Input: dimensioned drawing with shaded views. Units: mm. Origin: part minimum x, y, z. Round coordinates to 2 decimals unless told otherwise and drop trailing zeros. Order: outer loops, then holes, each group sorted by start corner. A loop starts at its lowest first (then second) coordinate and runs counter-clockwise, first axis right, second up. Notation, with made-up numbers: M -13,36 L -9,36 A5 ccw -9,42 Z; hole C -22.5,4 d8. An arc over 180 degrees is marked long. Answer as CSV lines item,"result". Start each with the question number.
Item 1: First-contact query: P1, Ø12, axis at y = 8.5, z = 10, coming from the +X side (1 decimal); P2, Ø10, axis at y = 16.5, z = 12, coming from the +X side (1 decimal); P3, Ø1, axis at y = 31, z = 19, coming from the -X side; P4, Ø10, axis at x = 8.5, y = 20.5, coming from the -Z side. Flat tips, straight axial feed; report the tip coordinate or a pass-through.
Item 2: Section query B-B on z = 18.5. Return the cut outline in (x, y) (1 decimal).
Item 3: Line query: line 1 (Y direction, x = 8.5, z = 23) (1 decimal); line 2 (Y direction, x = 9, z = 13.75); line 3 (Z direction, x = 12, y = 30.5) (1 decimal). Output: solid intervals per line, ascending. Write a range as [from, to].
Item 4: Pull-direction query (X, two-part tool) for the marked faces 1, 2 and 3; classes: +X half, -X half, draft (parallel to the pull), parting line (faces both ways), or undercut.
Item 5: Section query A-A on x = 12.75. Return the cut outline in (y, z).
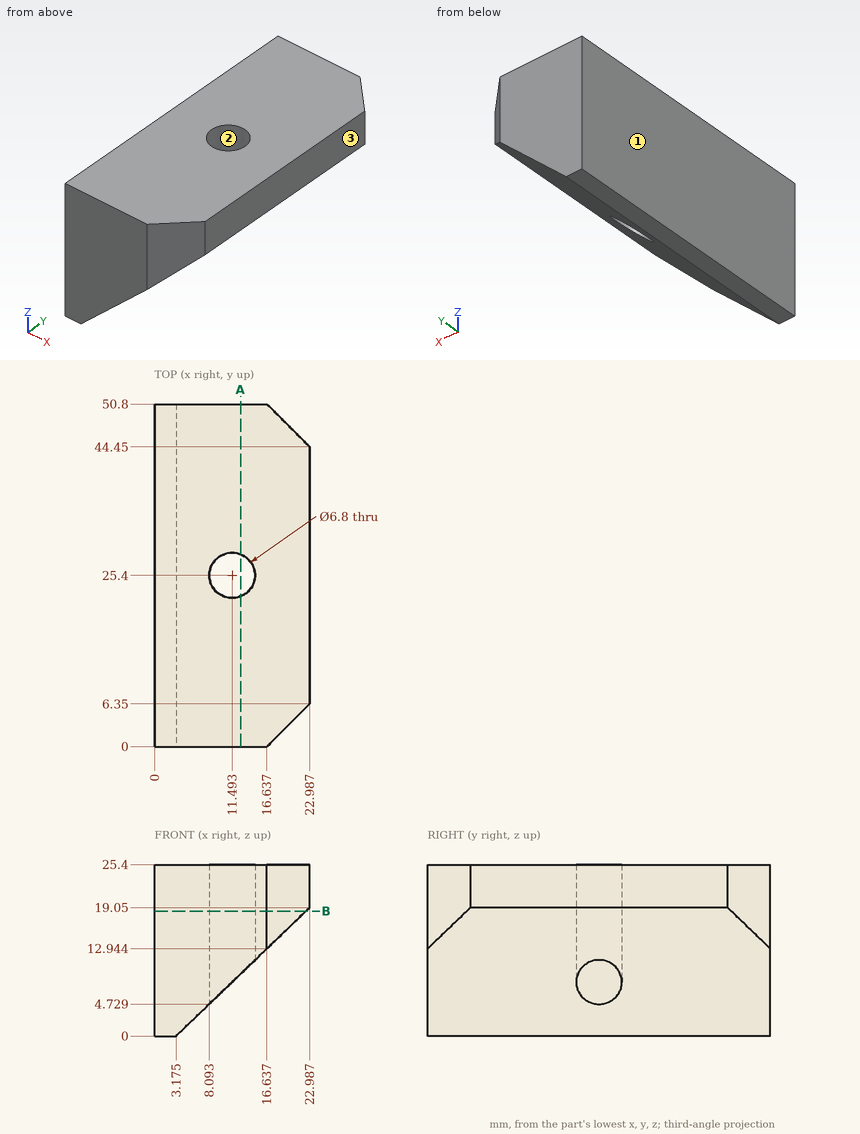
Results:
1,P1,"x = 19.8"
1,P2,"x = 20.9"
1,P3,"x = 0"
1,P4,"z = 0.31"
2,outline,"M 0,0 L 16.6,0 L 22.4,5.8 L 22.4,45 L 16.6,50.8 L 0,50.8 Z; hole C 11.5,25.4 d6.8"
3,line 1,"[0, 23.8], [27, 50.8]"
3,line 2,"[0, 23.09], [27.71, 50.8]"
3,line 3,"[8.5, 25.4]"
4,face 1,"-X half"
4,face 2,"undercut"
4,face 3,"+X half"
5,outline,"M 0,9.21 L 22.24,9.21 L 22.24,25.4 L 0,25.4 Z; M 28.56,9.21 L 50.8,9.21 L 50.8,25.4 L 28.56,25.4 Z"
